Could you check a few things on this model? Use its own coordinates, in mm. A direction names the side the tool comes from. Give positions to 0.01 mm unless a question says otherwise; leave off trailing zeros. Loops run counter-clockwise (first coordinate to the right, second up) from the corner with the lowest first, then second, coordinate; pieces in that order, holes last. Notation, with made-up numbers: (44.5, 79) - (81.5, 79) arc R22 ccw to (81.5, 87) - close; hole circle Ø4 at (67.5, 56). An arc over 180 degrees is marked (long way). Write each question's results on one line, items separated by ' | '. Start each with the question number.
(1) For pin 1 (4.5 mm diameter, centred on x = 2.5, y = 0, fed in from +Z); pin 2 (4.5 mm diameter, centred on y = 6.5, z = 2.5, fed in from +X); pin 3 (2 mm diameter, centred on x = 10, z = 3, fed in from +Y), each with a flat end and sliding along its axis, tell me the tip position at first contact or that it passes through.
(2) Suppose I cut it at C-C (z = 8). Please give me the cut outline in (x, y), and give its area (3 significant figures).
(3) Suppose I cut it at A-A (z = 5.25). Count the separate pieces of the cut face and the enclosed holes in it, and give its area (3 significant figures).
(4) Suppose I cut it at B-B (x = -14). Please give me the cut outline in (y, z), and give its area (3 significant figures).
(5) If we mould it in two halves opening along Z, with no side actions, what happens to faces 1 (the face through (-4.182, -1, 7)), 2 (the face through (-5.98, 7.77, 15.01)), 3 (the face through (7, -5, 14.5)), 4 (the face through (10, 0, 6))? For each: released by +Z, released by -Z, zero draft, split by the parting line, or undercut.
(6) Suppose I cut it at D-D (x = 15). Please give me the cut outline in (y, z), and give its area (4 significant figures).
(7) On a 3-axis mill with a long thin cutter (end or side, diameter ignored), from which of +Z, -Z, +X, -X, +Y, -Y can I reach the whole of each face in a straight line? I mean faces 5 (the face through (-8, 0, 0)), 6 (the face through (6.486, 0.477, 4.62)), 7 (the face through (4.426, 0.607, 11.049)), 8 (the face through (-1.672, 0.055, 6.757)). Say none if no direction works.
(8) I need wall thicknesses on line 1 (Y direction, x = 2.5, z = 14.8); line 2 (X direction, y = 0, z = 12.5); line 3 (X direction, y = 4.5, z = 2). Which ranges of each line are inside material? Lowest first, please.
from build123d import *

# Parameters (mm, degrees)
SKETCH1_W               = 35
SKETCH1_H               = 28
BOSS_EXTRUDE1_DEPTH     = 16
SKETCH2_R               = 11.5
CUT_EXTRUDE1_DEPTH      = 1.5
SKETCH3_R               = 2.0193
CUT_EXTRUDE2_DEPTH      = 7
SKETCH4_R               = 4.2164
CUT_EXTRUDE3_DEPTH      = 13.318
CUT_EXTRUDE4_REACH      = 32.366
CUT_EXTRUDE4_END_RADIUS = 2.0193
SKETCH5_R               = 1.2446
SKETCH6_R               = 6.5
SKETCH6_R_2             = 4.5
BOSS_EXTRUDE2_DEPTH     = 0.5
SKETCH7_R               = 0.5
CUT_EXTRUDE5_DEPTH      = 9
SKETCH15_W              = 15
SKETCH15_H              = 28
CUT_EXTRUDE9_DEPTH      = 6
SKETCH16_R              = 1.5875
SKETCH16_R_2            = 0.25
BOSS_EXTRUDE4_DEPTH     = 3
SKETCH17_R              = 0.515994608
SKETCH17_R_2            = 0.25
BOSS_EXTRUDE5_DEPTH     = 9
CHAMFER5_SIZE           = 0.5
CHAMFER6_SIZE           = 0.2
CHAMFER7_SIZE           = 0.5


with BuildPart() as part:
    # Sketch1 → Boss-Extrude1 (new body)
    with BuildSketch(Plane.XY):
        Rectangle(SKETCH1_W, SKETCH1_H)
    extrude(amount=BOSS_EXTRUDE1_DEPTH)

    # Sketch2 → Cut-Extrude1 (cut)
    with BuildSketch(Plane.XY.offset(16)):
        with Locations((2.5, 0)):
            Circle(SKETCH2_R)
    extrude(amount=-CUT_EXTRUDE1_DEPTH, mode=Mode.SUBTRACT)

    # Sketch3 → Cut-Extrude2 (cut)
    with BuildSketch(Plane.XY.offset(14.5)):
        with Locations((2.5, 0)):
            Circle(SKETCH3_R)
    extrude(amount=-CUT_EXTRUDE2_DEPTH, mode=Mode.SUBTRACT)

    # Sketch4 → Cut-Extrude3 (cut)
    with BuildSketch(Plane.ZY.offset(17.5)):
        with Locations((8, 0)):
            Circle(SKETCH4_R)
    extrude(amount=-CUT_EXTRUDE3_DEPTH, mode=Mode.SUBTRACT)

    # Cut-Extrude4: up to this cylinder (the profile starts outside it)
    cut_extrude4_end = Plane(origin=(2.5, 0, 8), z_dir=(0, 0, 1)) * Cylinder(CUT_EXTRUDE4_END_RADIUS, 69.7706, mode=Mode.PRIVATE)
    # Sketch5 → Cut-Extrude4 (cut, up to the surface)
    with BuildSketch(Plane.ZY.offset(4.182), mode=Mode.PRIVATE) as cut_extrude4_sk1:
        with Locations((8, 0)):
            Circle(SKETCH5_R)
    cut_extrude4_tool1 = extrude(cut_extrude4_sk1.sketch, amount=-CUT_EXTRUDE4_REACH, mode=Mode.PRIVATE) - cut_extrude4_end
    add(cut_extrude4_tool1.solids().sort_by_distance((-4.182, 0, 8))[0], mode=Mode.SUBTRACT)

    # Sketch6 → Boss-Extrude2 (add)
    with BuildSketch(Plane.XY.offset(14.5)):
        with Locations((2.5, 0)):
            Circle(SKETCH6_R)
        with Locations((2.5, 0)):
            Circle(SKETCH6_R_2, mode=Mode.SUBTRACT)
    extrude(amount=BOSS_EXTRUDE2_DEPTH)

    # Sketch7 → Cut-Extrude5 (cut)
    with BuildSketch(Plane.XY.offset(15)):
        with Locations((8, 0)):
            Circle(SKETCH7_R)
    extrude(amount=-CUT_EXTRUDE5_DEPTH, mode=Mode.SUBTRACT)

    # Sketch15 → Cut-Extrude9 (cut)
    with BuildSketch(Plane(origin=(0, 0, 0), x_dir=(-1, 0, 0), z_dir=(0, 0, -1))):
        with Locations((-10, 0)):
            Rectangle(SKETCH15_W, SKETCH15_H)
    extrude(amount=-CUT_EXTRUDE9_DEPTH, mode=Mode.SUBTRACT)

    # Sketch16 → Boss-Extrude4 (add)
    with BuildSketch(Plane(origin=(0, 0, 6), x_dir=(-1, 0, 0), z_dir=(0, 0, -1))):
        with Locations((-8, 0)):
            Circle(SKETCH16_R)
        with Locations((-8, 0)):
            Circle(SKETCH16_R_2, mode=Mode.SUBTRACT)
    extrude(amount=BOSS_EXTRUDE4_DEPTH)

    # Sketch17 → Boss-Extrude5 (add)
    with BuildSketch(Plane.XY.offset(6)):
        with Locations((8, 0)):
            Circle(SKETCH17_R)
        with Locations((8, 0)):
            Circle(SKETCH17_R_2, mode=Mode.SUBTRACT)
    extrude(amount=BOSS_EXTRUDE5_DEPTH)

    # Chamfer5
    chamfer5_edges = [part.edges().sort_by_distance(p)[0] for p in [
        (0, -14, 16),
        (-9, 0, 16),
        (17.5, 0, 16),
        (0, 14, 16),
        (-17.5, 0, 16),
    ]]
    chamfer(chamfer5_edges, length=CHAMFER5_SIZE)

    # Chamfer6
    chamfer6_edges = [part.edges().sort_by_distance(p)[0] for p in [
        (9.5875, 0, 3),
    ]]
    chamfer(chamfer6_edges, length=CHAMFER6_SIZE)

    # Chamfer7
    chamfer7_edges = [part.edges().sort_by_distance(p)[0] for p in [
        (-7.5, 14, 0),
        (-7.5, -14, 0),
        (10, -14, 6),
        (2.5, -14, 3),
        (17.5, 0, 6),
        (10, 14, 6),
        (2.5, 14, 3),
        (2.5, 0, 0),
        (-17.5, 0, 0),
        (17.5, 14, 10.75),
        (17.5, -14, 10.75),
        (-17.5, 14, 7.75),
        (-17.5, -14, 7.75),
    ]]
    chamfer(chamfer7_edges, length=CHAMFER7_SIZE)


solid = part.part
Output values:
1) pin 1: z = 14.5 | pin 2: x = 2.5 | pin 3: y = 1.22
2) outline: (-17.5, -13.5) - (-17, -14) - (17, -14) - (17.5, -13.5) - (17.5, 13.5) - (17, 14) - (-17, 14) - (-17.5, 13.5) - (-17.5, 4.22) - (-4.18, 4.22) - (-4.18, 1.24) - (0.91, 1.24) arc R2.02 cw (long way) to (0.91, -1.24) - (-4.18, -1.24) - (-4.18, -4.22) - (-17.5, -4.22) - close; hole circle Ø0.5 at (8, 0) | area: 842 mm2
3) separate pieces: 2 | enclosed holes: 1 | area: 482 mm2
4) outline: (-14, 0.5) - (-13.5, 0) - (13.5, 0) - (14, 0.5) - (14, 15.5) - (13.5, 16) - (-13.5, 16) - (-14, 15.5) - close; hole circle Ø8.43 at (0, 8) | area: 392 mm2
5) face 1: undercut | face 2: zero draft | face 3: released by +Z | face 4: released by -Z
6) outline: (-14, 6.5) - (-13.5, 6) - (13.5, 6) - (14, 6.5) - (14, 15.5) - (13.5, 16) - (-13.5, 16) - (-14, 15.5) - close | area: 279.5 mm2
7) face 5: -Z, +X, -X, +Y, -Y | face 6: -Z | face 7: +Z | face 8: -X
8) line 1: -14 to -11.5, -6.5 to -4.5, 4.5 to 6.5, 11.5 to 14 | line 2: -17.5 to 0.48, 4.52 to 7.75, 8.25 to 17.5 | line 3: -17.5 to 2.5
